```python
from build123d import *

# Parameters (mm, degrees)
CROQUIS1_R              = 1.5
CROQUIS1_R_2            = 6
SALIENTE_EXTRUIR1_DEPTH = 3
CROQUIS3_R              = 2
CORTAR_EXTRUIR1_DEPTH   = 10
CROQUIS4_R              = 5
CORTAR_EXTRUIR2_DEPTH   = 5
CROQUIS5_R              = 2.5
CORTAR_EXTRUIR3_DEPTH   = 10


with BuildPart() as part:
    # Croquis1 → Saliente-Extruir1 (new body)
    with BuildSketch(Plane.XY):
        with BuildLine():
            Line((207, -38), (-207, -38))
            ThreePointArc((-207, -38), (-228.213203436, -29.213203436), (-237, -8))
            Line((-237, -8), (-237, 16))
            ThreePointArc((-237, 16), (-228.213203436, 37.213203436), (-207, 46))
            Line((-207, 46), (207, 46))
            ThreePointArc((207, 46), (228.213203436, 37.213203436), (237, 16))
            Line((237, 16), (237, -8))
            ThreePointArc((237, -8), (228.213203436, -29.213203436), (207, -38))
        make_face()
        with Locations((15.5, 4)):
            Circle(CROQUIS1_R, mode=Mode.SUBTRACT)
        with Locations((7.496094703, -9.863170633)):
            Circle(CROQUIS1_R, mode=Mode.SUBTRACT)
        with Locations((-8.51171589, -9.863170633)):
            Circle(CROQUIS1_R, mode=Mode.SUBTRACT)
        with Locations((-16.515621187, 4)):
            Circle(CROQUIS1_R, mode=Mode.SUBTRACT)
        with Locations((-8.51171589, 17.863170633)):
            Circle(CROQUIS1_R, mode=Mode.SUBTRACT)
        with Locations((7.496094703, 17.863170633)):
            Circle(CROQUIS1_R, mode=Mode.SUBTRACT)
        with Locations((0, -3)):
            Circle(CROQUIS1_R_2, mode=Mode.SUBTRACT)
    extrude(amount=SALIENTE_EXTRUIR1_DEPTH)

    # Croquis3 → Cortar-Extruir1 (cut)
    with BuildSketch(Plane.XY.offset(3)):
        with Locations((-176.510078636, 20.458426503)):
            Circle(CROQUIS3_R)
        with Locations((-144.510078636, 20.458426503)):
            Circle(CROQUIS3_R)
        with Locations((-176.510078636, -11.541573497)):
            Circle(CROQUIS3_R)
        with Locations((-144.510078636, -11.541573497)):
            Circle(CROQUIS3_R)
        with Locations((-84.510078636, -11.541573497)):
            Circle(CROQUIS3_R)
        with Locations((-52.510078636, -11.541573497)):
            Circle(CROQUIS3_R)
        with Locations((-84.510078636, 20.458426503)):
            Circle(CROQUIS3_R)
        with Locations((-52.510078636, 20.458426503)):
            Circle(CROQUIS3_R)
        with BuildLine():
            Line((-171.81353386, -11.541573497), (-149.206623412, -11.541573497))
            ThreePointArc((-149.206623412, -11.541573497), (-146.967629564, -9.696790667), (-145.025631601, -7.541573497))
            Line((-145.025631601, -7.541573497), (-160.510078636, -7.541573497))
            Line((-160.510078636, -7.541573497), (-175.850570995, -7.725062086))
            ThreePointArc((-175.850570995, -7.725062086), (-173.968028908, -9.777151268), (-171.81353386, -11.541573497))
        make_face()
        with BuildLine():
            Line((-160.510078636, 8.458426503), (-141.332797807, 8.458426503))
            ThreePointArc((-141.332797807, 8.458426503), (-141.023531592, 6.469044388), (-140.920078636, 4.458426503))
            Line((-140.920078636, 4.458426503), (-180.100078636, 4.458426503))
            ThreePointArc((-180.100078636, 4.458426503), (-179.996625681, 6.469044388), (-179.687359465, 8.458426503))
            Line((-179.687359465, 8.458426503), (-160.510078636, 8.458426503))
        make_face()
        with BuildLine():
            Line((-160.510078636, 12.458426503), (-142.628017793, 12.458426503))
            ThreePointArc((-142.628017793, 12.458426503), (-143.707371652, 14.53002707), (-145.025631601, 16.458426503))
            Line((-145.025631601, 16.458426503), (-160.510078636, 16.458426503))
            Line((-160.510078636, 16.458426503), (-175.850570995, 16.641915092))
            ThreePointArc((-175.850570995, 16.641915092), (-177.252536774, 14.629866691), (-178.392139479, 12.458426503))
            Line((-178.392139479, 12.458426503), (-160.510078636, 12.458426503))
        make_face()
        with BuildLine():
            Line((-160.510078636, 0.458426503), (-141.332797807, 0.458426503))
            ThreePointArc((-141.332797807, 0.458426503), (-141.872785343, -1.576422186), (-142.628017793, -3.541573497))
            Line((-142.628017793, -3.541573497), (-160.510078636, -3.541573497))
            Line((-160.510078636, -3.541573497), (-178.392139479, -3.541573497))
            ThreePointArc((-178.392139479, -3.541573497), (-179.147371929, -1.576422186), (-179.687359465, 0.458426503))
            Line((-179.687359465, 0.458426503), (-160.510078636, 0.458426503))
        make_face()
        with BuildLine():
            Line((-171.81353386, 20.458426503), (-149.206623412, 20.458426503))
            ThreePointArc((-149.206623412, 20.458426503), (-160.510078636, 24.048426503), (-171.81353386, 20.458426503))
        make_face()
        with BuildLine():
            Line((-57.206623412, 20.458426503), (-79.81353386, 20.458426503))
            ThreePointArc((-79.81353386, 20.458426503), (-68.510078636, 24.048426503), (-57.206623412, 20.458426503))
        make_face()
        with BuildLine():
            Line((-68.510078636, -7.541573497), (-53.169586278, -7.725062086))
            ThreePointArc((-53.169586278, -7.725062086), (-55.052128364, -9.777151268), (-57.206623412, -11.541573497))
            Line((-57.206623412, -11.541573497), (-79.81353386, -11.541573497))
            ThreePointArc((-79.81353386, -11.541573497), (-82.052527708, -9.696790667), (-83.994525672, -7.541573497))
            Line((-83.994525672, -7.541573497), (-68.510078636, -7.541573497))
        make_face()
        with BuildLine():
            Line((-68.510078636, -3.541573497), (-50.628017793, -3.541573497))
            ThreePointArc((-50.628017793, -3.541573497), (-49.872785343, -1.576422186), (-49.332797807, 0.458426503))
            Line((-49.332797807, 0.458426503), (-68.510078636, 0.458426503))
            Line((-68.510078636, 0.458426503), (-87.687359465, 0.458426503))
            ThreePointArc((-87.687359465, 0.458426503), (-87.147371929, -1.576422186), (-86.392139479, -3.541573497))
            Line((-86.392139479, -3.541573497), (-68.510078636, -3.541573497))
        make_face()
        with BuildLine():
            Line((-68.510078636, 16.458426503), (-53.169586278, 16.641915092))
            ThreePointArc((-53.169586278, 16.641915092), (-51.767620498, 14.629866691), (-50.628017793, 12.458426503))
            Line((-50.628017793, 12.458426503), (-68.510078636, 12.458426503))
            Line((-68.510078636, 12.458426503), (-86.392139479, 12.458426503))
            ThreePointArc((-86.392139479, 12.458426503), (-85.312785621, 14.53002707), (-83.994525672, 16.458426503))
            Line((-83.994525672, 16.458426503), (-68.510078636, 16.458426503))
        make_face()
        with BuildLine():
            Line((-68.510078636, 8.458426503), (-49.332797807, 8.458426503))
            ThreePointArc((-49.332797807, 8.458426503), (-49.023531592, 6.469044388), (-48.920078636, 4.458426503))
            Line((-48.920078636, 4.458426503), (-88.100078636, 4.458426503))
            ThreePointArc((-88.100078636, 4.458426503), (-87.996625681, 6.469044388), (-87.687359465, 8.458426503))
            Line((-87.687359465, 8.458426503), (-68.510078636, 8.458426503))
        make_face()
    extrude(amount=-CORTAR_EXTRUIR1_DEPTH, mode=Mode.SUBTRACT)

    # Croquis4 → Cortar-Extruir2 (cut)
    with BuildSketch(Plane.XY.offset(3)):
        with Locations((-36.9, 4)):
            Circle(CROQUIS4_R)
    extrude(amount=-CORTAR_EXTRUIR2_DEPTH, mode=Mode.SUBTRACT)

    # Croquis5 → Cortar-Extruir3 (cut)
    with BuildSketch(Plane(origin=(0, 0, 0), x_dir=(-1, 0, 0), z_dir=(0, 0, -1))):
        with Locations((69, 33)):
            Circle(CROQUIS5_R)
        with Locations((161, 33)):
            Circle(CROQUIS5_R)
        with Locations(Location((161, -25, 0), (0, 0, 180))):
            Circle(CROQUIS5_R)
        with Locations(Location((69, -25, 0), (0, 0, 180))):
            Circle(CROQUIS5_R)
        with Locations((-69, -25)):
            Circle(CROQUIS5_R)
        with Locations((-161, -25)):
            Circle(CROQUIS5_R)
        with Locations(Location((-161, 33, 0), (0, 0, 180))):
            Circle(CROQUIS5_R)
        with Locations(Location((-69, 33, 0), (0, 0, 180))):
            Circle(CROQUIS5_R)
    extrude(amount=-CORTAR_EXTRUIR3_DEPTH, mode=Mode.SUBTRACT)


solid = part.part
```
The model under review builds one solid part; all positions refer to its coordinate system, in mm. Round coordinates to 2 decimals unless told otherwise and drop trailing zeros. Order: outer loops, then holes, each group sorted by start corner. A loop starts at its lowest first (then second) coordinate and runs counter-clockwise, first axis right, second up.
(1) Wall thickness on L1, parallel to X at y = 1, z = 1; L2, parallel to X at y = 17, z = 1.4; L3, parallel to X at y = -13, z = 2.6: over which ranges is each line inside the solid? List them lowest first.
Working result:
L1: x = -237 to -40.9, -32.9 to -4.47, 4.47 to 237
L2: x = -236.98 to -9.74, -7.28 to 6.27, 8.72 to 236.98
L3: x = -236.58 to -177.88, -175.14 to -145.88, -143.14 to -85.88, -83.14 to -53.88, -51.14 to 236.58
(2) For P1, Ø2.5, axis at x = -8.51, y = -9.86, coming from the +Z side, flat-tipped, find the tip position at first contact; note if it passes through.
Working result:
P1: passes through
(3) Take a section at A-A, the plane z = 2.3. Count the separate pieces of the cut face and the enclosed holes in it, plus the area to 3 significant figures.
Working result:
separate pieces: 1
enclosed holes: 34
area: 37,300 mm2
(4) Take a section at B-B, the plane y = -32.5. State the section outline as (x, z) points, plus the area to 3 significant figures.
Working result:
outline: (-224.31, 0) - (224.31, 0) - (224.31, 3) - (-224.31, 3) - close
area: 1,350 mm2
(5) Mouldability with a two-part tool opening along X and no side actions: class faces 1 (the face through (-6, -3, 1)), 2 (the face through (3, 5, 0)), 3 (the face through (-228.445, 36.979, 1.479)) as released by +X, released by -X, zero draft, split by the parting line, or undercut.
Working result:
face 1: undercut
face 2: zero draft
face 3: released by -X
